from build123d import *

# Parameters (mm, degrees)
SKETCH2_R           = 8.5
BOSS_EXTRUDE1_DEPTH = 5


with BuildPart() as part:
    # Sketch2 → Boss-Extrude1 (new body)
    with BuildSketch(Plane.XY):
        Polygon((0, 31), (0, 25), (5, 25), (5, 5), (0, 5), (0, 0), (10, 0), (10, -5), (30, -5), (30, 0), (50, 0), (50, -5), (70, -5), (70, 0), (80, 0), (80, 5), (75, 5), (75, 25), (80, 25), (80, 31), (70, 31), (70, 36), (50, 36), (50, 31), align=None)
        with Locations((41, 14.5)):
            Circle(SKETCH2_R, mode=Mode.SUBTRACT)
        with Locations((60, 14.5)):
            Circle(SKETCH2_R, mode=Mode.SUBTRACT)
    extrude(amount=-BOSS_EXTRUDE1_DEPTH)


solid = part.part
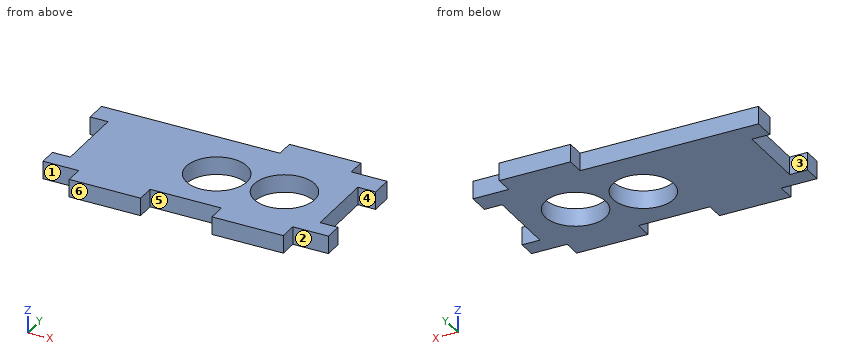
Source: CAD feature listing. Evaluate the final solid. Frame: model axes, mm. Face numbers are marked on the shaded views. A direction names the side the tool comes from. Give positions to 0.01 mm unless a question says otherwise; leave off trailing zeros. Write each loop counter-clockwise with the first axis right and the second up, starting at its lowest first coordinate (ties: lowest second). Pieces come first, ordered by that corner, then holes. Notation, with made-up numbers: (58.5, -17.5) -> (90.5, -17.5) arc R22 cw to (90.5, 4.5) -> close; hole circle Ø6 at (63, 22). An arc over 180 degrees is marked (long way). Return JSON: item names as keys, results as strings. Group by question number.
1. Section C-C, the plane y = 20. Output: boundary loops of the cut face in (x, z), then the cut area to 3 significant figures.
2. Material intervals for line 1 (Y direction, x = 60, z = -2.8); line 2 (Y direction, x = 41, z = -1.55); line 3 (X direction, y = 10, z = -4.65), sorted ascending. Write a range as from..to.
3. Section B-B, the plane z = -4. Output: boundary loops of the cut face in (x, y), then the cut area to 3 significant figures.
4. Pin query (flat end, axial travel): pin 1 Ø2.5 at (y, z) = (14, -2) entering from -X; pin 2 Ø2.5 at (x, z) = (77.5, -3.5) entering from +Y; pin 3 Ø1.5 at (x, z) = (76.5, -1.5) entering from -Y. Return the tip coordinate at first contact, or that it passes through.
5. Mould query, pull axis X, two halves, no side actions, for the marked faces 5 and 6. Classes: +X half, -X half, draft (parallel to the pull), parting line (faces both ways), or undercut.
6. Section A-A, the plane x = 41. Output: boundary loops of the cut face in (y, z), then the cut area to 3 significant figures.
7. Section D-D, the plane x = 60. Output: boundary loops of the cut face in (y, z), then the cut area to 3 significant figures.
8. Access query for the marked faces 1, 2, 3 and 4. Directions: +Z, -Z, +X, -X, +Y, -Y. A direction counts if a zero-diameter tool reaches every point of the face in a straight line with its end or side. Return the directions, or none.
Determined:
{
 "1": {"outline": "(5, -5) -> (34.52, -5) -> (34.52, 0) -> (5, 0) -> close; (47.48, -5) -> (53.52, -5) -> (53.52, 0) -> (47.48, 0) -> close; (66.48, -5) -> (75, -5) -> (75, 0) -> (66.48, 0) -> close", "area": "220 mm2"},
 "2": {"line 1": "y = -5..6, 23..36", "line 2": "y = 0..6, 23..31", "line 3": "x = 5..33.79, 48.21..52.79, 67.21..75"},
 "3": {"outline": "(0, 0) -> (10, 0) -> (10, -5) -> (30, -5) -> (30, 0) -> (50, 0) -> (50, -5) -> (70, -5) -> (70, 0) -> (80, 0) -> (80, 5) -> (75, 5) -> (75, 25) -> (80, 25) -> (80, 31) -> (70, 31) -> (70, 36) -> (50, 36) -> (50, 31) -> (0, 31) -> (0, 25) -> (5, 25) -> (5, 5) -> (0, 5) -> close; hole circle Ø17 at (41, 14.5); hole circle Ø17 at (60, 14.5)", "area": "2,130 mm2"},
 "4": {"pin 1": "stops at x = 5", "pin 2": "stops at y = 31", "pin 3": "stops at y = 0"},
 "5": {"face 5": "undercut", "face 6": "draft"},
 "6": {"outline": "(0, -5) -> (6, -5) -> (6, 0) -> (0, 0) -> close; (23, -5) -> (31, -5) -> (31, 0) -> (23, 0) -> close", "area": "70.0 mm2"},
 "7": {"outline": "(-5, -5) -> (6, -5) -> (6, 0) -> (-5, 0) -> close; (23, -5) -> (36, -5) -> (36, 0) -> (23, 0) -> close", "area": "120 mm2"},
 "8": {"face 1": "+Z, -Z, -X, -Y", "face 2": "+Z, -Z, +X, -Y", "face 3": "+Z, -Z, -X", "face 4": "+Z, -Z, +X"}
}
